from build123d import *

# Parameters (mm, degrees)
SKETCH1_R           = 101.6
BOSS_EXTRUDE1_DEPTH = 3.175
CUT_EXTRUDE3_DEPTH  = 1.5875
SKETCH3_R           = 14.224
CUT_EXTRUDE4_DEPTH  = 4.175


with BuildPart() as part:
    # Sketch1 → Boss-Extrude1 (new body)
    with BuildSketch(Plane.XY):
        Circle(SKETCH1_R)
    extrude(amount=BOSS_EXTRUDE1_DEPTH)

    # Sketch2 → Cut-Extrude3 (cut)
    with BuildSketch(Plane(origin=(0, 0, 0), x_dir=(-1, 0, 0), z_dir=(0, 0, -1))):
        with BuildLine():
            ThreePointArc((-88.771189624, -49.418983121), (-87.988181024, -50.8), (-87.183689624, -52.168613778))
            Line((-87.183689624, -52.168613778), (-1.5875, -2.749630657))
            Line((-1.5875, -2.749630657), (-1.5875, -0.916543552))
            Line((-1.5875, -0.916543552), (-3.175, 0))
            Line((-3.175, 0), (-88.771189624, -49.418983121))
        make_face()
        Polygon((-1.5875, -0.916543552), (-1.5875, -2.749630657), (0, -1.833087105), align=None)
        Polygon((-1.5875, -0.916543552), (0, -1.833087105), (1.5875, -0.916543552), (1.5875, 0.916543552), (0, 1.833087105), (-1.5875, 0.916543552), align=None)
        Polygon((1.5875, -0.916543552), (0, -1.833087105), (1.5875, -2.749630657), align=None)
        Polygon((-3.175, 0), (-1.5875, -0.916543552), (-1.5875, 0.916543552), align=None)
        Polygon((-1.5875, 2.749630657), (-1.5875, 0.916543552), (0, 1.833087105), align=None)
        Polygon((0, 1.833087105), (1.5875, 0.916543552), (1.5875, 2.749630657), align=None)
        Polygon((1.5875, 0.916543552), (1.5875, -0.916543552), (3.175, 0), align=None)
        with BuildLine():
            Line((1.5875, 0.916543552), (3.175, 0))
            Line((3.175, 0), (88.771189624, 49.418983121))
            ThreePointArc((88.771189624, 49.418983121), (87.988181024, 50.8), (87.183689624, 52.168613778))
            Line((87.183689624, 52.168613778), (1.5875, 2.749630657))
            Line((1.5875, 2.749630657), (1.5875, 0.916543552))
        make_face()
        with BuildLine():
            Line((3.175, 0), (1.5875, -0.916543552))
            Line((1.5875, -0.916543552), (1.5875, -2.749630657))
            Line((1.5875, -2.749630657), (87.183689624, -52.168613778))
            ThreePointArc((87.183689624, -52.168613778), (87.988181024, -50.8), (88.771189624, -49.418983121))
            Line((88.771189624, -49.418983121), (3.175, 0))
        make_face()
        with BuildLine():
            Line((-1.5875, 2.749630657), (0, 1.833087105))
            Line((0, 1.833087105), (1.5875, 2.749630657))
            Line((1.5875, 2.749630657), (1.5875, 101.587596899))
            ThreePointArc((1.5875, 101.587596899), (0, 101.6), (-1.5875, 101.587596899))
            Line((-1.5875, 101.587596899), (-1.5875, 2.749630657))
        make_face()
        with BuildLine():
            Line((-88.771189624, 49.418983121), (-3.175, 0))
            Line((-3.175, 0), (-1.5875, 0.916543552))
            Line((-1.5875, 0.916543552), (-1.5875, 2.749630657))
            Line((-1.5875, 2.749630657), (-87.183689624, 52.168613778))
            ThreePointArc((-87.183689624, 52.168613778), (-87.988181024, 50.8), (-88.771189624, 49.418983121))
        make_face()
        with BuildLine():
            Line((0, -1.833087105), (-1.5875, -2.749630657))
            Line((-1.5875, -2.749630657), (-1.5875, -101.587596899))
            ThreePointArc((-1.5875, -101.587596899), (0, -101.6), (1.5875, -101.587596899))
            Line((1.5875, -101.587596899), (1.5875, -2.749630657))
            Line((1.5875, -2.749630657), (0, -1.833087105))
        make_face()
    extrude(amount=-CUT_EXTRUDE3_DEPTH, mode=Mode.SUBTRACT)

    # Sketch3 → Cut-Extrude4 (cut, through all)
    with BuildSketch(Plane.XY.offset(3.175)):
        Circle(SKETCH3_R)
    extrude(amount=-CUT_EXTRUDE4_DEPTH, mode=Mode.SUBTRACT)


solid = part.part
Can you work these out from the model? Positions are in its coordinate system, mm. A direction names the side the tool comes from. Give positions to 0.01 mm unless a question says otherwise; leave off trailing zeros. Loops run counter-clockwise (first coordinate to the right, second up) from the corner with the lowest first, then second, coordinate; pieces in that order, holes last. Notation, with made-up numbers: (-36.5, 21.5) -> (-0.5, 21.5) arc R34 cw to (-0.5, 56.5) -> close; hole circle Ø8 at (-1.75, 11.25). An arc over 180 degrees is marked (long way). Write item = value, one per line.
1) Suppose I cut it at B-B on z = 2.25. Write out the boundary of the cut face in (x, y), then the cut area to 3 significant figures.
Check result:
outline = circle Ø203.2 at (0, 0); hole circle Ø28.45 at (0, 0)
area = 31,800 mm2
2) Suppose I cut it at C-C on x = 40. Write out the boundary of the cut face in (y, z) (1 decimal), then the cut area to 3 significant figures.
Check result:
outline = (-93.4, 0) -> (-24.9, 0) -> (-24.9, 1.6) -> (-21.3, 1.6) -> (-21.3, 0) -> (21.3, 0) -> (21.3, 1.6) -> (24.9, 1.6) -> (24.9, 0) -> (93.4, 0) -> (93.4, 3.2) -> (-93.4, 3.2) -> close
area = 581 mm2
3) Suppose I cut it at A-A on y = 0. Write out the boundary of the cut face in (x, z) (3 decimals), then the cut area to 3 significant figures.
Check result:
outline = (-101.6, 0) -> (-14.224, 0) -> (-14.224, 3.175) -> (-101.6, 3.175) -> close; (14.224, 0) -> (101.6, 0) -> (101.6, 3.175) -> (14.224, 3.175) -> close
area = 555 mm2
4) Suppose I cut it at D-D on y = -59. Write out the boundary of the cut face in (x, z) (1 decimal).
Check result:
outline = (-82.7, 0) -> (-1.6, 0) -> (-1.6, 1.6) -> (1.6, 1.6) -> (1.6, 0) -> (82.7, 0) -> (82.7, 3.2) -> (-82.7, 3.2) -> close
5) Will these pins go through, and if not, where does the flat tip stop? pin 1 (10 mm diameter, centred on x = -39.5, y = 31.5, fed in from -Z); pin 2 (1.5 mm diameter, centred on y = 78, z = 2, fed in from -X); pin 3 (0.5 mm diameter, centred on y = 52, z = 1, fed in from +X); pin 4 (0.8 mm diameter, centred on y = 44, z = 1, fed in from -X).
Check result:
pin_1 = 0
pin_2 = -65.99
pin_3 = 87.18
pin_4 = -91.77
6) Thinking about a two-plate mould opening in Y: for faces 3 (the flat face through (-68, 1, 0)), 4 (the cylindrical face through (-22.025, -99.184, 1.565)), 5 (the flat face through (50, 29, 1.588)), 6 (the flat face through (48.79, 30, 0.78)), which applies, released by +Y, released by -Y, zero draft, split by the parting line, or undercut?
Check result:
face_3 = zero draft
face_4 = split by the parting line
face_5 = undercut
face_6 = undercut
7) I need wall thicknesses on L1, parallel to Y at x = 38.5, z = 1.35; L2, parallel to Y at x = 45.5, z = 1.5; L3, parallel to Y at x = 0, z = 2.4. Which ranges of each line are inside material? Lowest first, please. Write a range as from..to.
Check result:
L1 = -94.02..-24.06, -20.39..20.39, 24.06..94.02
L2 = -90.84..-28.1, -24.44..24.44, 28.1..90.84
L3 = -101.6..-14.22, 14.22..101.6
8) For faces 1 (the flat face through (-49.846, 30.612, 0.783)), 2 (the flat face through (34, 56, 0)), which set-ups out of +Z, -Z, +X, -X, +Y, -Y let a thin tool reach every point of the face, with its end or its side?
Check result:
face_1 = -Z
face_2 = -Z, +X, -X, +Y, -Y
